```python
from build123d import *

# Parameters (mm, degrees)
SKETCH1_W               = 40
SKETCH1_H               = 40
BOSS_EXTRUDE1_DEPTH     = 40
CUT_EXTRUDE1_DEPTH      = 61
CUT_EXTRUDE1_DEPTH_BACK = 61
CUT_EXTRUDE2_DEPTH      = 61
CUT_EXTRUDE2_DEPTH_BACK = 35
SKETCH4_W               = 35
SKETCH4_H               = 35
CUT_EXTRUDE3_DEPTH      = 57.789083458
CUT_EXTRUDE3_DEPTH_BACK = 57.789083458
SKETCH6_R               = 4
CUT_EXTRUDE4_DEPTH      = 46
CUT_EXTRUDE4_DEPTH_BACK = 46
SKETCH5_R               = 4


with BuildPart() as part:
    # Sketch1 → Boss-Extrude1 (new body)
    with BuildSketch(Plane(origin=(0, 0, 0), x_dir=(1, 0, 0), z_dir=(0, 1, 0))):
        Rectangle(SKETCH1_W, SKETCH1_H)
    extrude(amount=BOSS_EXTRUDE1_DEPTH)

    # Sketch2 → Cut-Extrude1 (cut, two sides: drawn at the far end of the back side and taken through both)
    with BuildSketch(Plane(origin=(20, 0, 0), x_dir=(0, 0, -1), z_dir=(1, 0, 0)).offset(-CUT_EXTRUDE1_DEPTH_BACK)):
        Polygon((15, 40), (-20, 5), (-20, 40), align=None)
    extrude(amount=CUT_EXTRUDE1_DEPTH + CUT_EXTRUDE1_DEPTH_BACK, mode=Mode.SUBTRACT)

    # Sketch4 → Cut-Extrude2 (cut, two sides: drawn at the far end of the back side and taken through both)
    with BuildSketch(Plane.XY.offset(20).offset(-CUT_EXTRUDE2_DEPTH_BACK)):
        with Locations((0, 22.5)):
            Rectangle(SKETCH4_W, SKETCH4_H)
    extrude(amount=CUT_EXTRUDE2_DEPTH + CUT_EXTRUDE2_DEPTH_BACK, mode=Mode.SUBTRACT)

    # Sketch6 → Cut-Extrude3 (cut, two sides: drawn at the far end of the back side and taken through both)
    with BuildSketch(Plane.XY.offset(-15).offset(-CUT_EXTRUDE3_DEPTH_BACK)):
        with Locations((0, 20)):
            Circle(SKETCH6_R)
    extrude(amount=CUT_EXTRUDE3_DEPTH + CUT_EXTRUDE3_DEPTH_BACK, mode=Mode.SUBTRACT)

    # Sketch5 → Cut-Extrude4 (cut, two sides: drawn at the far end of the back side and taken through both)
    with BuildSketch(Plane(origin=(0, 5, 0), x_dir=(1, 0, 0), z_dir=(0, 1, 0)).offset(-CUT_EXTRUDE4_DEPTH_BACK)):
        with Locations(Location((0, 0, 0), (0, 0, 270))):
            Circle(SKETCH5_R)
    extrude(amount=CUT_EXTRUDE4_DEPTH + CUT_EXTRUDE4_DEPTH_BACK, mode=Mode.SUBTRACT)


solid = part.part
```
Here's how the part is built. I have some questions about the finished solid (model axes, mm). A direction names the side the tool comes from. Round coordinates to 2 decimals unless told otherwise and drop trailing zeros. Write each loop counter-clockwise with the first axis right and the second up, starting at its lowest first coordinate (ties: lowest second). Pieces come first, ordered by that corner, then holes.
Q1. If we mould it in two halves opening along X, with no side actions, what happens to faces 1 (the flat face through (-20, 15, -4)), 2 (the flat face through (20, 15, -4)), 3 (the flat face through (17.5, 18, -2)), 4 (the flat face through (-0.3, 24.2, -20))? For each: +X half, -X half, draft (parallel to the pull), parting line (faces both ways), or undercut.
Q2. Please list where these lines run through material, in increasing order: probe 1 along Z at (x, y) = (0, 1); probe 2 along X at (y, z) = (10.5, -7); probe 3 along Y at (x, z) = (0, -16).
Q3. If we section it at C-C on y = 20: Write out the boundary of the cut face in (x, z).
Q4. If we section it at B-B on z = 0: Write out the boundary of the cut face in (x, y).
Q5. Will these pins go through, and if not, where does the flat tip stop? P1, Ø1, axis at x = 7.5, y = 9.5, coming from the +Z side; P2, Ø1.5, axis at x = -15, z = 0, coming from the +Y side.
Q6. Which directions (+Z, -Z, +X, -X, +Y, -Y) give clear straight access to the entire face, cutting with the end or side of a thin tool? Please do faces 5 (the cylindrical face through (-0.521, 23.966, -17.535)), 6 (the flat face through (0, 27, -15)).
Q7. If we section it at D-D on z = -9.5: Write out the boundary of the cut face in (x, y).
Q8. If we section it at A-A on x = 0: Write out the boundary of the cut face in (y, z), plus the area to 3 significant figures.
Answer below:
1. face 1: -X half
1. face 2: +X half
1. face 3: undercut
1. face 4: draft
2. probe 1: z = -20 to -4, 4 to 20
2. probe 2: x = -20 to -17.5, 17.5 to 20
2. probe 3: y = 0 to 16, 24 to 40
3. outline: (-20, -20) - (-4, -20) - (-4, -15) - (-17.5, -15) - (-17.5, 5) - (-20, 5) - close; (4, -20) - (20, -20) - (20, 5) - (17.5, 5) - (17.5, -15) - (4, -15) - close
4. outline: (-20, 0) - (-4, 0) - (-4, 5) - (-17.5, 5) - (-17.5, 25) - (-20, 25) - close; (4, 0) - (20, 0) - (20, 25) - (17.5, 25) - (17.5, 5) - (4, 5) - close
5. P1: stops at z = -15
5. P2: stops at y = 5
6. face 5: +Z, -Z
6. face 6: +Z, +Y
7. outline: (-20, 0) - (20, 0) - (20, 34.5) - (17.5, 34.5) - (17.5, 5) - (-17.5, 5) - (-17.5, 34.5) - (-20, 34.5) - close
8. outline: (0, -20) - (16, -20) - (16, -15) - (5, -15) - (5, -4) - (0, -4) - close; (0, 4) - (5, 4) - (5, 20) - (0, 20) - close; (24, -20) - (40, -20) - (40, -15) - (24, -15) - close
8. area: 295 mm2
